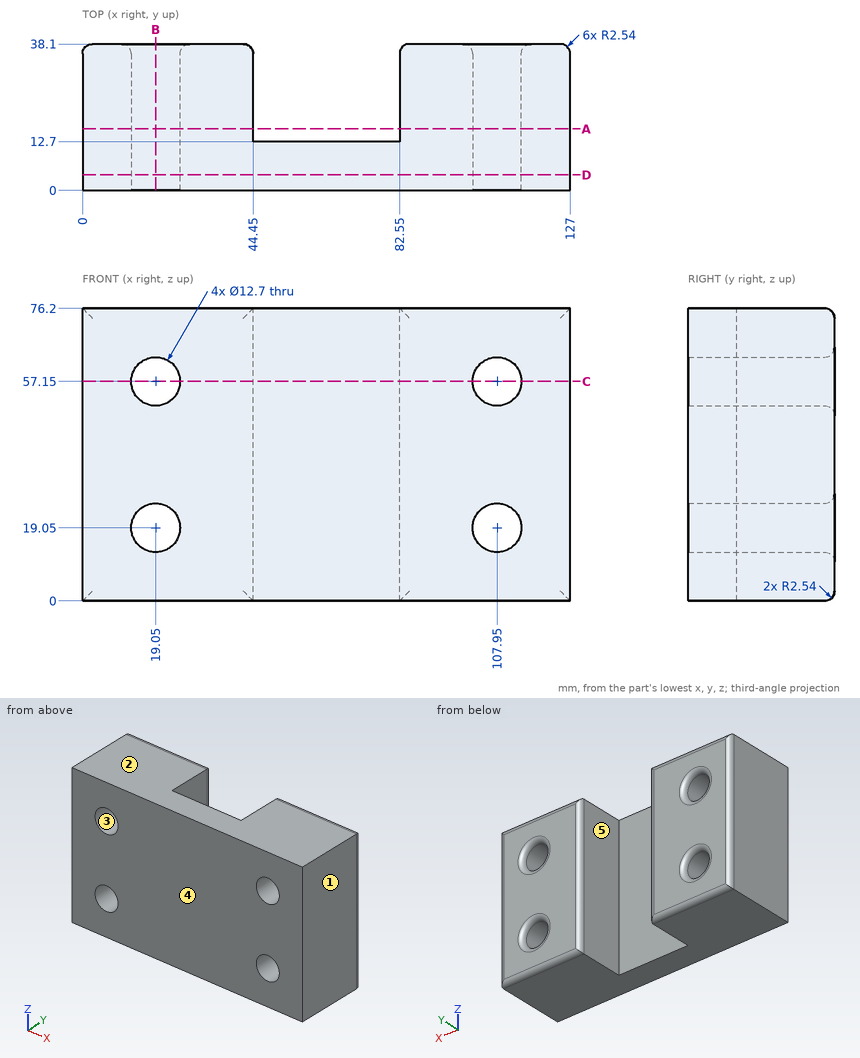
Check sheet for the drawn part. Datum: minimum x, y, z corner. Units: mm. A direction names the side the tool comes from. Give positions to 0.01 mm unless a question says otherwise; leave off trailing zeros. Order: outer loops, then holes, each group sorted by start corner. A loop starts at its lowest first (then second) coordinate and runs counter-clockwise, first axis right, second up. Notation, with made-up numbers: (72.5, 7.5) - (110.5, 7.5) arc R32 ccw to (110.5, 46.5) - close; hole circle Ø2 at (64, 61). An arc over 180 degrees is marked (long way). Write item = value, one per line. Start each with the question number.
1) Scan lines: L1, parallel to Z at x = 107.95, y = 27; L2, parallel to X at y = 19, z = 10; L3, parallel to X at y = 2.5, z = 58.5. Record each from-to range of solid material in increasing order.
2) Access from +Z, -Z, +X, -X, +Y, -Y to the whole of each face (thin tool, end or side, straight path). Record for the marked faces 4 and 5.
3) Section check C-C (z = 57.15). Enter the section's corners in (x, y).
4) Gauge pin test, flat ends, axial feed: pin 1 Ø4 at (x, z) = (57.5, 24.5) entering from +Y; pin 2 Ø16.5 at (x, z) = (19.05, 57.15) entering from +Y; pin 3 Ø10 at (x, y) = (66, 18.5) entering from +Z. Record the tip position at first contact, or that the pin passes through.
5) Draft check along X on the marked faces 1, 2 and 3. Enter one of: released by +X, released by -X, zero draft, split by the parting line, or undercut.
6) Section check B-B (x = 19.05). Enter the section's corners in (y, z).
7) Section check D-D (y = 4). Enter the section's corners in (x, z).
8) Section check A-A (y = 16). Enter the section's corners in (x, z), then the cut area to 3 significant figures.
Geometry check:
q1.L1 = 0 to 12.7, 25.4 to 50.8, 63.5 to 76.2
q1.L2 = 0 to 44.45, 82.55 to 127
q1.L3 = 0 to 12.85, 25.25 to 101.75, 114.15 to 127
q2.face_4 = +Z, -Z, +X, -X, -Y
q2.face_5 = +Z, -Z, +Y
q3.outline = (0, 0) - (12.7, 0) - (12.7, 35.56) arc R2.54 ccw to (10.16, 38.1) - (2.54, 38.1) arc R2.54 ccw to (0, 35.56) - close; (25.4, 0) - (101.6, 0) - (101.6, 35.56) arc R2.54 ccw to (99.06, 38.1) - (85.09, 38.1) arc R2.54 ccw to (82.55, 35.56) - (82.55, 12.7) - (44.45, 12.7) - (44.45, 35.56) arc R2.54 ccw to (41.91, 38.1) - (27.94, 38.1) arc R2.54 ccw to (25.4, 35.56) - close; (114.3, 0) - (127, 0) - (127, 35.56) arc R2.54 ccw to (124.46, 38.1) - (116.84, 38.1) arc R2.54 ccw to (114.3, 35.56) - close
q4.pin_1 = 12.7
q4.pin_2 = 38.02
q4.pin_3 = through
q5.face_1 = released by +X
q5.face_2 = zero draft
q5.face_3 = undercut
q6.outline = (0, 0) - (35.56, 0) arc R2.54 ccw to (38.1, 2.54) - (38.1, 10.16) arc R2.54 ccw to (35.56, 12.7) - (0, 12.7) - close; (0, 25.4) - (35.56, 25.4) arc R2.54 ccw to (38.1, 27.94) - (38.1, 48.26) arc R2.54 ccw to (35.56, 50.8) - (0, 50.8) - close; (0, 63.5) - (35.56, 63.5) arc R2.54 ccw to (38.1, 66.04) - (38.1, 73.66) arc R2.54 ccw to (35.56, 76.2) - (0, 76.2) - close
q7.outline = (0, 0) - (127, 0) - (127, 76.2) - (0, 76.2) - close; hole circle Ø12.7 at (19.05, 19.05); hole circle Ø12.7 at (19.05, 57.15); hole circle Ø12.7 at (107.95, 19.05); hole circle Ø12.7 at (107.95, 57.15)
q8.outline = (0, 0) - (44.45, 0) - (44.45, 76.2) - (0, 76.2) - close; (82.55, 0) - (127, 0) - (127, 76.2) - (82.55, 76.2) - close; hole circle Ø12.7 at (19.05, 19.05); hole circle Ø12.7 at (19.05, 57.15); hole circle Ø12.7 at (107.95, 19.05); hole circle Ø12.7 at (107.95, 57.15)
q8.area = 6,270 mm2
